Autodesk Inventor part; units mm, degrees
ref_plane "YZ Plane" through (0, 0, 0) normal (1, 0, 0) x (0, 1, 0)
ref_plane "XZ Plane" through (0, 0, 0) normal (0, 1, 0) x (-1, 0, 0)
ref_plane "XY Plane" through (0, 0, 0) normal (0, 0, 1) x (1, 0, 0)
sketch "Sketch1" plane through (0, 0, 0) normal (0, 0, 1) x (1, 0, 0)
  line L0 (20.5, 37.5) -> (51.5, 37.5) construction
  line L1 (51.5, 37.5) -> (51.5, 6.5) construction
  line L2 (51.5, 6.5) -> (20.5, 6.5) construction
  line L3 (20.5, 6.5) -> (20.5, 37.5) construction
  line L4 (14.62, 43.38) -> (57.38, 43.38) construction
  line L5 (57.38, 43.38) -> (57.38, 0.62) construction
  line L6 (57.38, 0.62) -> (14.62, 0.62) construction
  line L7 (14.62, 0.62) -> (14.62, 43.38) construction
  circle A0 centre (20.5, 6.5) radius 1.6
  circle A1 centre (51.5, 6.5) radius 1.6
  circle A2 centre (51.5, 37.5) radius 1.6
  circle A3 centre (20.5, 37.5) radius 1.6
  circle A4 centre (36, 22) radius 11.5
  circle A5 centre (13, 22) radius 4 construction
  circle A6 centre (7, 6) radius 2.25
  circle A7 centre (80.75, 49.5) radius 2.25
  line L8 (2, 56) -> (86.75, 56)
  line L9 (88.75, 54) -> (88.75, 2)
  line L10 (86.75, 0) -> (2, 0)
  line L11 (0, 2) -> (0, 54)
  line L12 (0, 2) -> (2, 0)
  line L13 (0, 54) -> (2, 56)
  line L14 (86.75, 56) -> (88.75, 54)
  line L15 (88.75, 2) -> (86.75, 0)
  circle A8 centre (7, 6) radius 4.5 construction
  circle A9 centre (80.75, 49.5) radius 4.5 construction
  point P0 (0, 0)
  point P1 (36, 37.5)
  point P2 (51.5, 22)
  point P3 (14.62, 22)
  point P4 (36, 43.38)
  point P5 (0, 56)
  point P6 (88.75, 0)
  point P7 (88.75, 56)
  point P8 (0, 0)
  dimension "d0" = 31
  dimension "d1" = 42.76
  dimension "d2" = 3.2
  dimension "d3" = 23
  dimension "d4" = 8
  dimension "d5" = 23
  dimension "d6" = 4.5
  dimension "d7" = 2
  dimension "d8" = 2
  dimension "d9" = 2
  dimension "d10" = 2
  dimension "d11" = 2
  dimension "d12" = 2
  dimension "d13" = 2
  dimension "d14" = 2
  dimension "d15" = 22
  dimension "d16" = 9
  dimension "d17" = 6
  dimension "d18" = 6
  dimension "d19" = 29.25
  dimension "d20" = 12
  dimension "d22" = 36
  dimension "d23" = 34
  dimension "d26" = 8
extrude "Extrusion1" add sketch "Sketch1" along normal blind 6.5
properties part number "z_rod_stopper_bottom" material "Plywood, Finish"
The listing builds one solid part. Answer for the finished solid, in the listing's coordinates (mm). Round coordinates to 2 decimals unless told otherwise and drop trailing zeros. Loops run counter-clockwise (first coordinate to the right, second up) from the corner with the lowest first, then second, coordinate; pieces in that order, holes last.
Q1. For a pull along X with two mould halves and no side action, classify faces 1 (the face through (45, 0, 3)), 2 (the face through (52.98, 7.11, 3.2)), 3 (the face through (1, 55, 3)), 4 (the face through (87.74, 55.01, 3.2)) as released by +X, released by -X, zero draft, split by the parting line, or undercut.
Q2. Section C-C, the plane z = 5.5 is taken. Determine the outline of the cut face in (x, y).
Q3. Find the intervals of material crossed by line 1 (Y direction, x = 20.5, z = 3); line 2 (Y direction, x = 7, z = 5); line 3 (X direction, y = 7, z = 2.5), in increasing order.
Q4. Section B-B, the plane y = 49.5 is taken. Determine the outline of the cut face in (x, z).
Q5. Given pin 1 Ø3.5 at (x, y) = (80.75, 49.5) entering from +Z, flat-ended and moving along its own axis, determine where the tip first touches the part or whether it passes through.
Q6. Section D-D, the plane y = 37.5 is taken. Determine the outline of the cut face in (x, z), then the cut area to 3 significant figures.
Q7. Section A-A, the plane x = 20.5 is taken. Determine the outline of the cut face in (y, z).
Completed:
1. face 1: zero draft
1. face 2: undercut
1. face 3: released by -X
1. face 4: released by +X
2. outline: (0, 2) - (2, 0) - (86.75, 0) - (88.75, 2) - (88.75, 54) - (86.75, 56) - (2, 56) - (0, 54) - close; hole circle Ø4.5 at (7, 6); hole circle Ø3.2 at (20.5, 6.5); hole circle Ø3.2 at (20.5, 37.5); hole circle Ø23 at (36, 22); hole circle Ø3.2 at (51.5, 6.5); hole circle Ø3.2 at (51.5, 37.5); hole circle Ø4.5 at (80.75, 49.5)
3. line 1: y = 0 to 4.9, 8.1 to 35.9, 39.1 to 56
3. line 2: y = 0 to 3.75, 8.25 to 56
3. line 3: x = 0 to 4.98, 9.02 to 18.98, 22.02 to 49.98, 53.02 to 88.75
4. outline: (0, 0) - (78.5, 0) - (78.5, 6.5) - (0, 6.5) - close; (83, 0) - (88.75, 0) - (88.75, 6.5) - (83, 6.5) - close
5. pin 1: passes through
6. outline: (0, 0) - (18.9, 0) - (18.9, 6.5) - (0, 6.5) - close; (22.1, 0) - (49.9, 0) - (49.9, 6.5) - (22.1, 6.5) - close; (53.1, 0) - (88.75, 0) - (88.75, 6.5) - (53.1, 6.5) - close
6. area: 535 mm2
7. outline: (0, 0) - (4.9, 0) - (4.9, 6.5) - (0, 6.5) - close; (8.1, 0) - (35.9, 0) - (35.9, 6.5) - (8.1, 6.5) - close; (39.1, 0) - (56, 0) - (56, 6.5) - (39.1, 6.5) - close
